from build123d import *

# Parameters (mm, degrees)
CROQUIS1_R                 = 4.825
SALIENTE_EXTRUIR1_DEPTH    = 9
CROQUIS2_R                 = 2.53
SALIENTE_EXTRUIR2_DEPTH    = 200
CROQUIS3_R                 = 4.825
CORTAR_EXTRUIR1_DEPTH      = 29
CORTAR_EXTRUIR1_DEPTH_BACK = 67


with BuildPart() as part:
    # Croquis1 → Saliente-Extruir1 (new body)
    with BuildSketch(Plane(origin=(0, 0, 0), x_dir=(1, 0, 0), z_dir=(0, 1, 0))):
        Polygon((14.68670308, 0), (7.34335154, 12.719057965), (-7.34335154, 12.719057965), (-14.68670308, 0), (-7.34335154, -12.719057965), (7.34335154, -12.719057965), align=None)
        Circle(CROQUIS1_R, mode=Mode.SUBTRACT)
    extrude(amount=SALIENTE_EXTRUIR1_DEPTH)

    # Croquis2 → Saliente-Extruir2 (add)
    with BuildSketch(Plane.XY):
        with Locations((0, 4.5)):
            Circle(CROQUIS2_R)
    extrude(amount=SALIENTE_EXTRUIR2_DEPTH)

    # Croquis3 → Cortar-Extruir1 (cut, two sides)
    with BuildSketch(Plane(origin=(0, 0, 0), x_dir=(1, 0, 0), z_dir=(0, 1, 0))) as cortar_extruir1_sk:
        Circle(CROQUIS3_R)
    extrude(amount=CORTAR_EXTRUIR1_DEPTH, mode=Mode.SUBTRACT)
    extrude(cortar_extruir1_sk.sketch, amount=-CORTAR_EXTRUIR1_DEPTH_BACK, mode=Mode.SUBTRACT)


solid = part.part
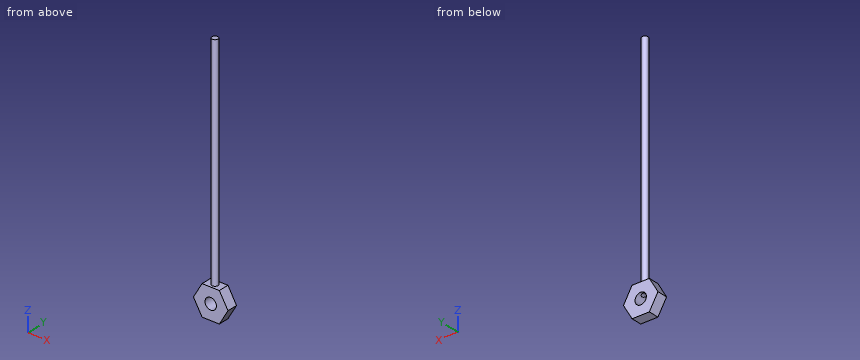
Build history of the part. All positions in model axes, mm. Give positions to 0.01 mm unless a question says otherwise; leave off trailing zeros. Order: outer loops, then holes, each group sorted by start corner. A loop starts at its lowest first (then second) coordinate and runs counter-clockwise, first axis right, second up. Notation, with made-up numbers: M -23.5,69 L -4.5,69 A29 cw -4.5,99 Z; hole C 30.25,79 d9. An arc over 180 degrees is marked long. Put each result on its own line as item: value.
Item 1: Slice it at C-C, the plane x = -9.25. Write the cut outline in (y, z).
From the geometry:
outline: M 0,-9.42 L 9,-9.42 L 9,9.42 L 0,9.42 Z
Item 2: Flat gauge pins, fed straight in: pin 1 Ø1.5 at (y, z) = (6.5, 170.5) entering from +X; pin 2 Ø3 at (x, z) = (1, 44) entering from +Y; pin 3 Ø3 at (y, z) = (4, 140.5) entering from +X. Where does each tip first touch, or does it go through?
From the geometry:
pin 1: stops at x = 2.2
pin 2: stops at y = 7.03
pin 3: stops at x = 2.53
Item 3: Probe line 1 (X direction, y = 5.25, z = 0) (3 decimals); line 2 (Z direction, x = 0, y = 4.75) (3 decimals); line 3 (Z direction, x = 3.75, y = 8). List the from-to ranges inside material, lowest first. Write a range as [from, to].
From the geometry:
line 1: x = [-14.687, -4.825], [4.825, 14.687]
line 2: z = [-12.719, -4.825], [4.825, 200]
line 3: z = [-12.72, -3.04], [3.04, 12.72]
Item 4: Slice it at B-B, the plane z = 102. Write the cut outline in (x, y).
From the geometry:
outline: C 0,4.5 d5.06
Item 5: Slice it at A-A, the plane x = 0. Write the cut outline in (y, z) (3 decimals), plus the area to 3 significant figures.
From the geometry:
outline: M 0,-12.719 L 9,-12.719 L 9,-4.825 L 0,-4.825 Z; M 0,4.825 L 9,4.825 L 9,12.719 L 7.03,12.719 L 7.03,200 L 1.97,200 L 1.97,12.719 L 0,12.719 Z
area: 1,090 mm2
